Could you check a few things on this model? Use its own coordinates, in mm. A direction names the side the tool comes from. Coordinates: 2 decimals unless noted, no trailing zeros. Write each loop counter-clockwise with the first axis right and the second up, starting at its lowest first coordinate (ties: lowest second). Pieces come first, ordered by that corner, then holes. Notation, with made-up numbers: (-31.5, -32) - (-16.5, -32) arc R33 ccw to (-16.5, -2) - close; hole circle Ø7 at (7, -28). An arc over 180 degrees is marked (long way). Answer as a JSON object with one key per item and string values. Group by question number.
1) If we section it at C-C (z = 6.25): Write out the boundary of the cut face in (x, y).
2) Will these pins go through, and if not, where does the flat tip stop? pin 1 Ø1.2 at (y, z) = (3.5, 2.5) entering from -X; pin 2 Ø1.7 at (x, z) = (0.5, 5.5) entering from -Y; pin 3 Ø2.5 at (x, y) = (0.5, 3.5) entering from -Z.
3) Please list where these lines run through material, in increasing order: line 1 along Y through (x, z) = (0, 4.25); line 2 along Z through (x, y) = (0, 5.6); line 3 along Y through (x, z) = (2.25, 3).
4) If we section it at B-B (y = 0.5): Write out the boundary of the cut face in (x, z).
5) We'd pull the mould along Y, two halves only. Please class faces 1 (the flat face through (0.04, 4.8, 3.75)), 2 (the flat face through (-7.396, -4.19, 2.218)), 3 (the cylindrical face through (1.526, 6.624, 2.481)): released by +Y, released by -Y, zero draft, split by the parting line, or undercut.
6) If we section it at D-D (z = 2): Write out the boundary of the cut face in (x, y), plus the area to 3 significant figures.
7) If we section it at A-A (x = 0): Write out the boundary of the cut face in (y, z), plus the area to 3 significant figures.
8) On a 3-axis mill with a long thin cutter (end or side, diameter ignored), from which of +Z, -Z, +X, -X, +Y, -Y can I reach the whole of each face in a straight line? I mean faces 4 (the flat face through (0, 2.5, 6)), 5 (the cylindrical face through (-6.094, 0.268, 6.472)), 6 (the flat face through (0, 4, 4)). Say none if no direction works.
```python
from build123d import *

# Parameters (mm, degrees)
SKETCH_R        = 3
PAD_DEPTH       = 4.5
SKETCH001_R     = 6.1
SKETCH001_R_2   = 3
PAD001_DEPTH    = 10
PAD002_DEPTH    = 13
SKETCH003_R     = 6.1
POCKET_DEPTH    = 6
PAD003_DEPTH    = 1.5
POCKET001_DEPTH = 4
SKETCH005_R     = 1.6
POCKET002_DEPTH = 3.701


with BuildPart() as part:
    # Sketch → Pad (new body)
    with BuildSketch(Plane.XY):
        Polygon((9.814955, 0), (4.907477, 8.5), (-4.907477, 8.5), (-9.814955, 0), (-4.907477, -8.5), (4.907477, -8.5), align=None)
        Circle(SKETCH_R, mode=Mode.SUBTRACT)
    extrude(amount=PAD_DEPTH)

    # Sketch001 (on Face9 of Pad) → Pad001 (join)
    with BuildSketch(Plane.XY.offset(4.5)):
        Circle(SKETCH001_R)
        Circle(SKETCH001_R_2, mode=Mode.SUBTRACT)
    extrude(amount=PAD001_DEPTH)

    # Sketch002 (on Face12 of Pad001) → Pad002 (join)
    with BuildSketch(Plane.XY.offset(14.5)):
        with BuildLine():
            Line((-1.658312, 2.5), (1.658312, 2.5))
            ThreePointArc((1.658312, 2.5), (0, 3), (-1.658312, 2.5))
        make_face()
    extrude(amount=-PAD002_DEPTH)

    # Sketch003 (on Face15 of Pad002) → Pocket (cut)
    with BuildSketch(Plane.XY.offset(14.5)):
        Circle(SKETCH003_R)
    extrude(amount=-POCKET_DEPTH, mode=Mode.SUBTRACT)

    # Pocket Face13 → Pad003 (add)
    with BuildSketch(Plane(origin=(0, 2.701501, 1.5), x_dir=(0, -1, 0), z_dir=(0, 0, -1))):
        with BuildLine():
            Line((0.201501, -1.658312), (0.201501, 1.658312))
            ThreePointArc((0.201501, 1.658312), (-0.298499, 0), (0.201501, -1.658312))
        make_face()
    extrude(amount=PAD003_DEPTH)

    # Sketch004 (on Face4 of Pad003) → Pocket001 (cut)
    with BuildSketch(Plane(origin=(0, 0, 0), x_dir=(1, 0, 0), z_dir=(0, 0, -1))):
        Polygon((2.8, -2.5), (2.8, -4.8), (-2.8, -4.8), (-2.8, -2.5), (0, -2.5), align=None)
    extrude(amount=-POCKET001_DEPTH, mode=Mode.SUBTRACT)

    # Sketch005 (on Face12 of Pocket001) → Pocket002 (cut, through all)
    with BuildSketch(Plane.XZ.offset(-4.8)):
        with Locations((0, 2)):
            Circle(SKETCH005_R)
    extrude(amount=-POCKET002_DEPTH, mode=Mode.SUBTRACT)


solid = part.part
```
Here are the results:
{
 "1": {"outline": "circle Ø12.2 at (0, 0); hole (-1.66, 2.5) arc R3 ccw (long way) to (1.66, 2.5) - close"},
 "2": {"pin 1": "stops at x = -8.14", "pin 2": "stops at y = -6.1", "pin 3": "stops at z = 4"},
 "3": {"line 1": "y = -8.5 to -3, 2.5 to 8.5", "line 2": "z = 0 to 0.4, 3.6 to 8.5", "line 3": "y = -8.5 to -1.98, 1.98 to 2.5, 4.8 to 8.5"},
 "4": {"outline": "(-9.53, 0) - (-2.96, 0) - (-2.96, 8.5) - (-6.08, 8.5) - (-6.08, 4.5) - (-9.53, 4.5) - close; (2.96, 0) - (9.53, 0) - (9.53, 4.5) - (6.08, 4.5) - (6.08, 8.5) - (2.96, 8.5) - close"},
 "5": {"face 1": "undercut", "face 2": "released by -Y", "face 3": "zero draft"},
 "6": {"outline": "(-9.81, 0) - (-4.91, -8.5) - (4.91, -8.5) - (9.81, 0) - (4.91, 8.5) - (1.6, 8.5) - (1.6, 4.8) - (2.8, 4.8) - (2.8, 2.5) - (1.66, 2.5) arc R3 cw (long way) to (-1.66, 2.5) - (-2.8, 2.5) - (-2.8, 4.8) - (-1.6, 4.8) - (-1.6, 8.5) - (-4.91, 8.5) - close", "area": "198 mm²"},
 "7": {"outline": "(-8.5, 0) - (-3, 0) - (-3, 8.5) - (-6.1, 8.5) - (-6.1, 4.5) - (-8.5, 4.5) - close; (2.5, 4) - (4.8, 4) - (4.8, 3.6) - (8.5, 3.6) - (8.5, 4.5) - (6.1, 4.5) - (6.1, 8.5) - (2.5, 8.5) - close; (4.8, 0) - (8.5, 0) - (8.5, 0.4) - (4.8, 0.4) - close", "area": "57.5 mm²"},
 "8": {"face 4": "+Z, -Z", "face 5": "+Z", "face 6": "-Z"}
}
